from build123d import *

# Parameters (mm, degrees)
F0_W     = 16.1053412664
F0_H     = 30.2006552678
F1_DEPTH = 44.704
F2_T     = -2.54
F3_DEPTH = 8.636
F5_DEPTH = 25.4


with BuildPart() as f1:
    # F0 (on Front) → F1 (new body)
    with BuildSketch(Plane.XZ):
        Polygon((-87.6387814232, 42.9285356432), (-103.7184670568, 61.1999630928), (-112.852960825, 52.5708459318), (-96.1492801466, 34.8888902675), align=None)
        Polygon((-80.0439388802, 34.8888902675), (-87.6387814232, 42.9285356432), (-96.1492801466, 34.8888902675), align=None)
        Polygon((-69.8299892996, 59.7520354048), (-87.6387814232, 42.9285356432), (-80.0439388802, 34.8888902675), (-62.3481592001, 51.8320212083), align=None)
        with Locations((-88.0966095134, 19.7885626337)):
            Rectangle(F0_W, F0_H)
    extrude(amount=F1_DEPTH)

    # F2
    f2_openings = [f1.faces().sort_by_distance(p)[0] for p in [
        (-104.50112, -22.352, 43.729868),
        (-96.14928, -22.352, 19.788563),
        (-80.043939, -22.352, 19.788563),
        (-71.196049, -22.352, 43.360456),
        (-95.678624, -22.352, 52.064249),
        (-78.734385, -22.352, 51.340286),
    ]]
    offset(amount=F2_T, openings=f2_openings)

    # F3 (add): a face of the model
    f3_faces = [f1.faces().sort_by_distance(p)[0] for p in [
        (-108.2857139409, -22.352, 56.8854045123),
    ]]
    extrude(f3_faces, amount=F3_DEPTH)

    # F4 (on face) → F5 (cut)
    with BuildSketch(Plane(origin=(-96.1492801466, 0, 0), x_dir=(0, -1, 0), z_dir=(-1, 0, 0))):
        with BuildLine():
            ThreePointArc((21.2460036068, 7.2282349998), (22.352, 6.1222386066), (23.4579963932, 7.2282349998))
            Line((23.4579963932, 7.2282349998), (21.2460036068, 7.2282349998))
        make_face()
    extrude(amount=-F5_DEPTH, mode=Mode.SUBTRACT)


solid = f1.part
The model under review builds one solid part; all positions refer to its coordinate system, in mm. A direction names the side the tool comes from. Give positions to 0.01 mm unless a question says otherwise; leave off trailing zeros. Order: outer loops, then holes, each group sorted by start corner. A loop starts at its lowest first (then second) coordinate and runs counter-clockwise, first axis right, second up. Notation, with made-up numbers: (53.25, 65) -> (87.25, 65) arc R9 ccw to (87.25, 78) -> close; hole circle Ø7 at (71, 32.5). An arc over 180 degrees is marked (long way). Write item = value, one per line. Start each with the question number.
(1) Take a section at D-D (x = -93.5). Write out the cut boundary in (y, z).
(2) Take a section at C-C (z = 46.5). Write out the cut boundary in (x, y), plus the area to 3 significant figures.
(3) Take a section at B-B (z = 28). Write out the cut boundary in (x, y).
(4) Draft analysis for pull direction Y (two halves, no side actions). For faces 6 (the flat face through (-96.149, -19, 6)), 7 (the flat face through (-67.88, -22.07, 53.99)), 8 (the flat face through (-89, -44.704, 38)), state which applies: +Y half, -Y half, draft (parallel to the pull), parting line (faces both ways), or undercut.
(5) For L1, parallel to Y at x = -81, z = 17.5; L2, parallel to Z at x = -83, y = -3; L3, parallel to X at y = -20, z = 57, list the stretches that pass through material, from the lowest coordinate up. Write a range as from..to.
(6) Tool access review of faces 1 (the flat face through (-88, -2.54, 34)), 2 (the flat face through (-80.044, -19, 6)), 3 (the flat face through (-88, -12, 7.228)), 4 (the flat face through (-102.192, -18.936, 59.466)), 5 (the flat face through (-106.51, -22.07, 55.07)): name each direction out of +Z, -Z, +X, -X, +Y, -Y from which nothing blocks a thin tool from reaching the whole face with its end or side.
(7) Take a section at A-A (y = -27). Write out the cut boundary in (x, z).
(8) For pin 1 Ø5 at (x, y) = (-90, -11.5) entering from +Z; pin 2 Ø12 at (y, z) = (-11.5, 38.5) entering from -X; pin 3 Ø3 at (x, y) = (-105, -20.5) entering from -Z, all flat-tipped, find the tip position at first contact; note any pin that passes through.
Returned:
q1.outline = (-44.7, 4.69) -> (0, 4.69) -> (0, 49.59) -> (-2.54, 49.59) -> (-2.54, 7.23) -> (-21.25, 7.23) arc R1.11 cw to (-23.46, 7.23) -> (-42.16, 7.23) -> (-42.16, 49.59) -> (-44.7, 49.59) -> close
q2.outline = (-107.12, -44.7) -> (-90.78, -44.7) -> (-90.78, -42.16) -> (-107.12, -42.16) -> close; (-107.12, -2.54) -> (-90.78, -2.54) -> (-90.78, 0) -> (-107.12, 0) -> close; (-83.86, -44.7) -> (-67.92, -44.7) -> (-67.92, -42.16) -> (-83.86, -42.16) -> close; (-83.86, -2.54) -> (-67.92, -2.54) -> (-67.92, 0) -> (-83.86, 0) -> close
q2.area = 164 mm²
q3.outline = (-96.15, -44.7) -> (-80.04, -44.7) -> (-80.04, -42.16) -> (-96.15, -42.16) -> close; (-96.15, -2.54) -> (-80.04, -2.54) -> (-80.04, 0) -> (-96.15, 0) -> close
q4.face_6 = draft
q4.face_7 = undercut
q4.face_8 = -Y half
q5.L1 = -44.7..-42.16, -2.54..0
q5.L2 = 4.69..7.23
q5.L3 = -117.04..-104.47, -70.72..-67.23
q6.face_1 = none
q6.face_2 = -Z, +X, +Y, -Y
q6.face_3 = +Z, +X, -X
q6.face_4 = +Z, +Y, -Y
q6.face_5 = -Z
q7.outline = (-118.78, 58.85) -> (-111.11, 50.72) -> (-102.04, 59.29) -> (-103.72, 61.2) -> (-109.65, 67.48) -> close; (-96.15, 4.69) -> (-80.04, 4.69) -> (-80.04, 7.23) -> (-96.15, 7.23) -> close; (-71.68, 58.01) -> (-64.18, 50.08) -> (-62.35, 51.83) -> (-69.83, 59.75) -> close
q8.pin_1 = 7.23
q8.pin_2 = through
q8.pin_3 = 55.08
